```python
from build123d import *

# Parameters (mm, degrees)
F0_W      = 15
F0_H      = 3
F1_DEPTH  = 2
F2_W      = 15
F2_H      = 10
F3_DEPTH  = 8
F4_R      = 2
F5_DEPTH  = 25
F6_R      = 4.99999
F7_W      = 15
F7_H      = 8
F7_H_2    = 2
F8_DEPTH  = 10
F9_R      = 4.99999
F10_R     = 2
F11_DEPTH = 25
F12_W     = 15
F12_H     = 2
F12_H_2   = 8
F13_DEPTH = 10
F14_R     = 4.99999
F15_R     = 2
F16_DEPTH = 25
F17_R     = 5


# Not quite as in the source:
# - a fillet or chamfer is up to 0.001 mm smaller than in the source, because OpenCascade refuses the exact size


with BuildPart() as f1:
    # F0 (on Top) → F1 (new body)
    with BuildSketch(Plane.XY):
        Polygon((0, 25), (-30, 5), (-15, 5), (-15, 2), (-15, -2), (-15, -5), (-30, -5), (0, -25), (0, -10), (-10, -10), (-10, 10), (0, 10), align=None)
        with Locations((-22.5, 3.5)):
            Rectangle(F0_W, F0_H)
        Polygon((-30, 2), (-30, 0), (-30, -2), (-15, -2), (-15, 2), align=None)
        with Locations((-22.5, -3.5)):
            Rectangle(F0_W, F0_H)
    extrude(amount=F1_DEPTH)

    # F2 (on face) → F3 (join)
    with BuildSketch(Plane.XY.offset(2)):
        with Locations((-22.5, 0)):
            Rectangle(F2_W, F2_H)
    extrude(amount=F3_DEPTH)

    # F4 (on face) → F5 (cut)
    with BuildSketch(Plane(origin=(-30, 0, 0), x_dir=(0, -1, 0), z_dir=(-1, 0, 0))):
        with Locations((0, 5)):
            Circle(F4_R)
    extrude(amount=-F5_DEPTH, mode=Mode.SUBTRACT)

    # F6 (radius 5 in the source; OpenCascade refuses exactly that, so slightly less here)
    f6_edges = [f1.edges().sort_by_distance(p)[0] for p in [
        (-22.5, -5, 10),
        (-22.5, 5, 10),
    ]]
    fillet(f6_edges, radius=F6_R)

    # F7 (on face) → F8 (join)
    with BuildSketch(Plane.YZ):
        with Locations((-17.5, 6)):
            Rectangle(F7_W, F7_H)
        with Locations((-17.5, 1)):
            Rectangle(F7_W, F7_H_2)
    extrude(amount=F8_DEPTH)

    # F9 (radius 5 in the source; OpenCascade refuses exactly that, so slightly less here)
    f9_edges = [f1.edges().sort_by_distance(p)[0] for p in [
        (0, -17.5, 10),
        (10, -17.5, 10),
        (10, -17.5, 0),
    ]]
    fillet(f9_edges, radius=F9_R)

    # F10 (on face) → F11 (cut)
    with BuildSketch(Plane.XZ.offset(25)):
        with Locations((5, 5)):
            Circle(F10_R)
    extrude(amount=-F11_DEPTH, mode=Mode.SUBTRACT)

    # F12 (on face) → F13 (join)
    with BuildSketch(Plane.YZ):
        with Locations((17.5, 1)):
            Rectangle(F12_W, F12_H)
        with Locations((17.5, 6)):
            Rectangle(F12_W, F12_H_2)
    extrude(amount=F13_DEPTH)

    # F14 (radius 5 in the source; OpenCascade refuses exactly that, so slightly less here)
    f14_edges = [f1.edges().sort_by_distance(p)[0] for p in [
        (0, 17.5, 10),
        (10, 17.5, 10),
        (10, 17.5, 0),
    ]]
    fillet(f14_edges, radius=F14_R)

    # F15 (on face) → F16 (cut)
    with BuildSketch(Plane(origin=(0, 25, 0), x_dir=(-1, 0, 0), z_dir=(0, 1, 0))):
        with Locations((-5, 5)):
            Circle(F15_R)
    extrude(amount=-F16_DEPTH, mode=Mode.SUBTRACT)

    # F17
    f17_edges = [f1.edges().sort_by_distance(p)[0] for p in [
        (-10, 10, 1),
        (-10, -10, 1),
    ]]
    fillet(f17_edges, radius=F17_R)


solid = f1.part
```
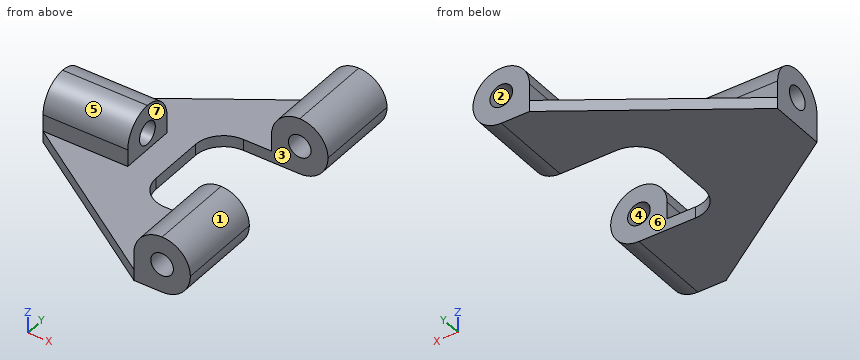
Geometry check sheet. Reference: the model listing, model coordinates, mm. Face numbers are marked on the shaded views. A direction names the side the tool comes from. Round coordinates to 2 decimals unless told otherwise and drop trailing zeros. Loops run counter-clockwise (first coordinate to the right, second up) from the corner with the lowest first, then second, coordinate; pieces in that order, holes last. Notation, with made-up numbers: (-10.75, -10.75) -> (45.25, -10.75) arc R10 ccw to (45.25, -3.75) -> close; hole circle Ø11 at (12, 70.25). An arc over 180 degrees is marked (long way). Use a Markdown table: item, result.
(1) Scan lines: probe 1 along Y at (x, z) = (6, 1.25); probe 2 along Z at (x, y) = (-25.5, 0); probe 3 along Y at (x, z) = (-20, 4.75). Record each from-to range of solid material in increasing order.
Calculated:
| item | result |
|---|---|
| probe 1 | -25 to -10, 10 to 25 |
| probe 2 | 0 to 3, 7 to 10 |
| probe 3 | -5 to -1.98, 1.98 to 5 |
(2) Sectioned sample at D-D (x = -7.5). Enter the section's corners in (y, z), then the cut area to 3 significant figures.
Calculated:
| item | result |
|---|---|
| outline | (-20, 0) -> (-9.33, 0) -> (-9.33, 2) -> (-20, 2) -> close; (9.33, 0) -> (20, 0) -> (20, 2) -> (9.33, 2) -> close |
| area | 42.7 mm² |
(3) Mould release check, pull along X, two halves, no side actions. Record for the marked faces 1, 2, 3 and 4: released by +X, released by -X, zero draft, split by the parting line, or undercut.
Calculated:
| item | result |
|---|---|
| face 1 | released by +X |
| face 2 | undercut |
| face 3 | zero draft |
| face 4 | undercut |
(4) Sectioned sample at C-C (z = 8.25). Enter the section's corners in (x, y), then the cut area to 3 significant figures.
Calculated:
| item | result |
|---|---|
| outline | (-30, -3.8) -> (-15, -3.8) -> (-15, 3.8) -> (-30, 3.8) -> close; (1.2, -25) -> (8.8, -25) -> (8.8, -10) -> (1.2, -10) -> close; (1.2, 10) -> (8.8, 10) -> (8.8, 25) -> (1.2, 25) -> close |
| area | 342 mm² |
(5) Go/stop test with flat-tipped pins: P1, Ø1, axis at y = 2, z = 1.5, coming from the +X side; P2, Ø5, axis at x = -7, z = 6.5, coming from the +Y side; P3, Ø15, axis at x = -14.5, y = 11.5, coming from the +Z side; P4, Ø1.5, axis at y = 16, z = 3.5, coming from the -X side. Record where each tip stops, or that it passes through.
Calculated:
| item | result |
|---|---|
| P1 | x = -10 |
| P2 | through |
| P3 | z = 7.98 |
| P4 | x = 0 |
(6) Set-up check for the marked faces 5, 6 and 7: record each of +Z, -Z, +X, -X, +Y, -Y from which the full face is reachable in a straight line by a thin tool's end or side.
Calculated:
| item | result |
|---|---|
| face 5 | +Z, +X, -X, -Y |
| face 6 | +Z, -Z, +X |
| face 7 | +Z, +X, +Y, -Y |
